Check sheet for the modelled part. Datum: model origin and axes. Units: mm. Round coordinates to 2 decimals unless told otherwise and drop trailing zeros. Loops run counter-clockwise (first coordinate to the right, second up) from the corner with the lowest first, then second, coordinate; pieces in that order, holes last. Notation, with made-up numbers: (44.5, 88.5) - (84.5, 88.5) arc R15 ccw to (84.5, 116.5) - close; hole circle Ø3 at (53, 58.25). An arc over 180 degrees is marked (long way). Return JSON: item names as keys, results as strings.
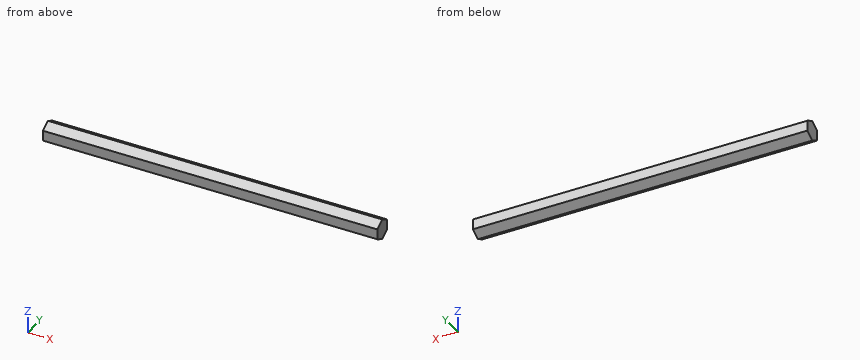
Autodesk Fusion 360 part; units mm, degrees
sketch "Sketch1" plane through (0, 0, 0) normal (1, 0, 0) x (0, 1, 0)
  line L0 (150, 45.3) -> (154.0703, 47.65)
  line L1 (154.0703, 47.65) -> (154.0703, 52.35)
  line L2 (154.0703, 52.35) -> (150, 54.7)
  line L3 (150, 54.7) -> (145.9297, 52.35)
  line L4 (145.9297, 52.35) -> (145.9297, 47.65)
  line L5 (145.9297, 47.65) -> (150, 45.3)
  point P0 (150, 50)
  dimension "d1" = 4.7
extrude "Extrude1" add sketch "Sketch1" against normal blind 150
Q1. Depth check by flat-ended pin: P1, Ø3, axis at x = -41.5, y = 152, coming from the -Z side; P2, Ø2, axis at x = -103, y = 152, coming from the +Z side. Enter the tip coordinate at first touch or a pass-through.
Answer key:
{"P1": "stops at z = 45.59", "P2": "stops at z = 54.12"}
Q2. Sectioned sample at B-B (y = 152.5). Enter the section's corners in (x, z), plus the area to 3 significant figures.
Answer key:
{"outline": "(-150, 46.74) - (0, 46.74) - (0, 53.26) - (-150, 53.26) - close", "area": "977 mm²"}
Q3. Sectioned sample at A-A (x = -124.5). Enter the section's corners in (y, z), plus the area to 3 significant figures.
Answer key:
{"outline": "(145.93, 47.65) - (150, 45.3) - (154.07, 47.65) - (154.07, 52.35) - (150, 54.7) - (145.93, 52.35) - close", "area": "57.4 mm²"}
Q4. Scan lines: probe 1 along Z at (x, y) = (-54.5, 147.75); probe 2 along Z at (x, y) = (-57.5, 149.75); probe 3 along Y at (x, z) = (-130, 46). Record each from-to range of solid material in increasing order. Write a range as [from, to].
Answer key:
{"probe 1": "z = [46.6, 53.4]", "probe 2": "z = [45.44, 54.56]", "probe 3": "y = [148.79, 151.21]"}
